```python
from build123d import *

# Parameters (mm, degrees)
BOSS_EXTRUDE1_DEPTH  = 1
SKETCH2_W            = 16
SKETCH2_H            = 10
BOSS_EXTRUDE2_DEPTH  = 10
SKETCH3_W            = 4.889113018
SKETCH3_H            = 5.37802432
CUT_EXTRUDE1_DEPTH   = 10
SKETCH4_W            = 45
SKETCH4_H            = 2.4
SKETCH4_W_2          = 30
BOSS_EXTRUDE3_DEPTH  = 4
SKETCH5_W            = 35
SKETCH5_H            = 10
BOSS_EXTRUDE4_DEPTH  = 7
SKETCH6_W            = 35
SKETCH6_H            = 1.5
CUT_EXTRUDE2_DEPTH   = 4
FILLET1_R            = 1
SKETCH7_R            = 1.5
CUT_EXTRUDE3_DEPTH   = 4
SKETCH8_W            = 0.75
SKETCH8_H            = 0.75
BOSS_EXTRUDE5_DEPTH  = 6
LPATTERN1_COUNT      = 10
LPATTERN1_PITCH      = 3
SKETCH9_W            = 0.75
SKETCH9_H            = 0.75
BOSS_EXTRUDE6_DEPTH  = 6
LPATTERN2_COUNT      = 15
LPATTERN2_PITCH      = 3
SKETCH10_R           = 2.5
BOSS_EXTRUDE7_DEPTH  = 6
SKETCH11_W           = 4.8
SKETCH11_H           = 9
BOSS_EXTRUDE8_DEPTH  = 4
SKETCH12_W           = 0.75
SKETCH12_H           = 0.75
BOSS_EXTRUDE9_DEPTH  = 6
LPATTERN3_COUNT      = 3
LPATTERN3_PITCH      = 3
LPATTERN3_COUNT_DIR2 = 2
LPATTERN3_PITCH_DIR2 = 3
SKETCH13_W           = 14.120912951
SKETCH13_H           = 4.362558473
BOSS_EXTRUDE10_DEPTH = 4
FILLET2_R            = 1


with BuildPart() as part:
    # Sketch1 → Boss-Extrude1 (new body)
    with BuildSketch(Plane.XY):
        Polygon((22.754016647, 124.270947632), (19.754016647, 127.270947632), (-47.799898806, 127.270947632), (-47.799898806, 75.270947632), (19.754016647, 75.270947632), (19.754016647, 90.113910289), (22.754016647, 92.500164177), align=None)
    extrude(amount=-BOSS_EXTRUDE1_DEPTH)

    # Sketch2 → Boss-Extrude2 (add)
    with BuildSketch(Plane(origin=(0, 0, -1), x_dir=(-1, 0, 0), z_dir=(0, 0, -1))):
        with Locations((46.316496684, 91.208096568)):
            Rectangle(SKETCH2_W, SKETCH2_H)
    extrude(amount=BOSS_EXTRUDE2_DEPTH)

    # Sketch3 → Cut-Extrude1 (cut)
    with BuildSketch(Plane.ZY.offset(54.316496684)):
        with Locations((-6.06540843, 91.2419286)):
            Rectangle(SKETCH3_W, SKETCH3_H)
    extrude(amount=-CUT_EXTRUDE1_DEPTH, mode=Mode.SUBTRACT)

    # Sketch4 → Boss-Extrude3 (add)
    with BuildSketch(Plane(origin=(0, 0, -1), x_dir=(-1, 0, 0), z_dir=(0, 0, -1))):
        with Locations((5.745983353, 78.470947632)):
            Rectangle(SKETCH4_W, SKETCH4_H)
        with Locations((-0.254016647, 124.070947632)):
            Rectangle(SKETCH4_W_2, SKETCH4_H)
    extrude(amount=BOSS_EXTRUDE3_DEPTH)

    # Sketch5 → Boss-Extrude4 (add)
    with BuildSketch(Plane(origin=(0, 0, -1), x_dir=(-1, 0, 0), z_dir=(0, 0, -1))):
        with Locations((3.745983353, 113.370947632)):
            Rectangle(SKETCH5_W, SKETCH5_H)
    extrude(amount=BOSS_EXTRUDE4_DEPTH)

    # Sketch6 → Cut-Extrude2 (cut)
    with BuildSketch(Plane(origin=(0, 0, -8), x_dir=(-1, 0, 0), z_dir=(0, 0, -1))):
        with Locations((3.745983353, 117.620947632)):
            Rectangle(SKETCH6_W, SKETCH6_H)
        with Locations((3.745983353, 109.120947632)):
            Rectangle(SKETCH6_W, SKETCH6_H)
    extrude(amount=-CUT_EXTRUDE2_DEPTH, mode=Mode.SUBTRACT)

    # Fillet1
    fillet1_edges = [part.edges().sort_by_distance(p)[0] for p in [
        (13.754016647, 109.870947632, -6),
        (-21.245983353, 109.870947632, -6),
        (13.754016647, 116.870947632, -6),
        (-21.245983353, 116.870947632, -6),
    ]]
    fillet(fillet1_edges, radius=FILLET1_R)

    # Sketch7 → Cut-Extrude3 (cut)
    with BuildSketch(Plane(origin=(0, 0, -1), x_dir=(-1, 0, 0), z_dir=(0, 0, -1))):
        with Locations((-20.390504743, 123.506772987)):
            Circle(SKETCH7_R)
        with Locations((-20.390504743, 93.48031176)):
            Circle(SKETCH7_R)
        with Locations((31.799898806, 123.506772987)):
            Circle(SKETCH7_R)
        with Locations((31.799898806, 78.192140702)):
            Circle(SKETCH7_R)
    extrude(amount=-CUT_EXTRUDE3_DEPTH, mode=Mode.SUBTRACT)

    # Sketch8 → Boss-Extrude5 (add)
    with BuildSketch(Plane(origin=(0, 0, -5), x_dir=(-1, 0, 0), z_dir=(0, 0, -1))):
        with Locations((-13.879016647, 124.070947632)):
            Rectangle(SKETCH8_W, SKETCH8_H)
    boss_extrude5 = extrude(amount=BOSS_EXTRUDE5_DEPTH)

    # LPattern1: Boss-Extrude5 ×10
    with Locations(*[(-i * LPATTERN1_PITCH, 0, 0) for i in range(1, LPATTERN1_COUNT)]):
        add(boss_extrude5)

    # Sketch9 → Boss-Extrude6 (add)
    with BuildSketch(Plane(origin=(0, 0, -5), x_dir=(-1, 0, 0), z_dir=(0, 0, -1))):
        with Locations((-15.402792453, 78.470947632)):
            Rectangle(SKETCH9_W, SKETCH9_H)
    boss_extrude6 = extrude(amount=BOSS_EXTRUDE6_DEPTH)

    # LPattern2: Boss-Extrude6 ×15
    with Locations(*[(-i * LPATTERN2_PITCH, 0, 0) for i in range(1, LPATTERN2_COUNT)]):
        add(boss_extrude6)

    # Sketch10 → Boss-Extrude7 (add)
    with BuildSketch(Plane(origin=(0, 0, -1), x_dir=(-1, 0, 0), z_dir=(0, 0, -1))):
        with Locations(Location((26.546732083, 118.214976991, 0), (0, 0, 180))):
            Circle(SKETCH10_R)
        with Locations(Location((31.940661119, 118.214976991, 0), (0, 0, 180))):
            Circle(SKETCH10_R)
    extrude(amount=BOSS_EXTRUDE7_DEPTH)

    # Sketch11 → Boss-Extrude8 (add)
    with BuildSketch(Plane(origin=(0, 0, -1), x_dir=(-1, 0, 0), z_dir=(0, 0, -1))):
        with Locations((-19.349242758, 100.613910289)):
            Rectangle(SKETCH11_W, SKETCH11_H)
    extrude(amount=BOSS_EXTRUDE8_DEPTH)

    # Sketch12 → Boss-Extrude9 (add)
    with BuildSketch(Plane(origin=(0, 0, -5), x_dir=(-1, 0, 0), z_dir=(0, 0, -1))):
        with Locations((-20.624242758, 97.488910289)):
            Rectangle(SKETCH12_W, SKETCH12_H)
    boss_extrude9 = extrude(amount=BOSS_EXTRUDE9_DEPTH)

    # LPattern3: Boss-Extrude9 3 × 2
    with Locations(*[(-j * LPATTERN3_PITCH_DIR2, i * LPATTERN3_PITCH, 0) for i in range(LPATTERN3_COUNT) for j in range(LPATTERN3_COUNT_DIR2) if (i, j) != (0, 0)]):
        add(boss_extrude9)

    # Sketch13 → Boss-Extrude10 (add)
    with BuildSketch(Plane(origin=(0, 0, -1), x_dir=(-1, 0, 0), z_dir=(0, 0, -1))):
        with Locations((23.447660741, 101.747194556)):
            Rectangle(SKETCH13_W, SKETCH13_H)
    extrude(amount=BOSS_EXTRUDE10_DEPTH)

    # Fillet2
    fillet2_edges = [part.edges().sort_by_distance(p)[0] for p in [
        (-16.387204265, 103.928473792, -3),
        (-16.387204265, 99.565915319, -3),
        (-30.508117216, 99.565915319, -3),
        (-30.508117216, 103.928473792, -3),
    ]]
    fillet(fillet2_edges, radius=FILLET2_R)


solid = part.part
```
Check sheet for the modelled part. Datum: model origin and axes. Units: mm. A direction names the side the tool comes from. Round coordinates to 2 decimals unless told otherwise and drop trailing zeros. Order: outer loops, then holes, each group sorted by start corner. A loop starts at its lowest first (then second) coordinate and runs counter-clockwise, first axis right, second up. Notation, with made-up numbers: (21, 2) -> (52, 2) arc R31 cw to (52, 32) -> close; hole circle Ø8 at (47.25, -13.75). An arc over 180 degrees is marked (long way). Use CSV: the item, a comma, the result in double quotes.
(1) Draft check along Y on faces 4 (the face through (21.23, 91.29, -0.49)), 5 (the face through (-49, 93.931, -6)), 6 (the face through (-46, 91, -11)). Enter one of: pulls with the +Y half, pulls with the -Y half, needs draft (parallel to the pull), parting line crosses it, or undercut.
Worked out:
face 4,"pulls with the -Y half"
face 5,"undercut"
face 6,"needs draft"
(2) Cross-section at B-B (z = -2). Count the separate pieces of the cut face and the enclosed holes in it, and give its area (3 significant figures).
Worked out:
separate pieces,"8"
enclosed holes,"0"
area,"833 mm²"
(3) Depth check by flat-ended pin: pin 1 (2 mm diameter, centred on x = -28, z = -3, fed in from -Y); pin 2 (1.5 mm diameter, centred on y = 112, z = -7.5, fed in from -X); pin 3 (0.6 mm diameter, centred on x = 17.5, z = -9, fed in from +Y). Enter the tip coordinate at first touch or a pass-through.
Worked out:
pin 1,"y = 77.27"
pin 2,"x = -21.25"
pin 3,"y = 103.86"
(4) Material ranges on line 1 along Y through (x, z) = (-18.5, -1.75); line 2 along Y through (x, z) = (-27, -3.25); line 3 along X through (y, z) = (97.5, -8.75), recorded low to high. Write a range as from..to.
Worked out:
line 1,"77.27..79.67, 99.57..103.93, 108.37..118.37"
line 2,"77.27..79.67, 99.57..103.93, 115.76..120.67"
line 3,"17.25..18, 20.25..21"
(5) Tool access check on faces 1 (the face through (-23, 103.928, -3)), 2 (the face through (-4, 109.871, -6)), 3 (the face through (-28.246, 78, -3)). Record the directions out of +Z, -Z, +X, -X, +Y, -Y that give a thin tool (end or side, any length) a straight path to the whole face; none if there is none.
Worked out:
face 1,"-Z, -X"
face 2,"-Z, +X, -X"
face 3,"-Z, -X, -Y"
(6) Cross-section at A-A (x = -46). Record the boundary of the cut face in (y, z).
Worked out:
outline,"(75.27, -1) -> (86.21, -1) -> (86.21, -11) -> (96.21, -11) -> (96.21, -1) -> (127.27, -1) -> (127.27, 0) -> (75.27, 0) -> close; hole (88.55, -8.51) -> (93.93, -8.51) -> (93.93, -3.62) -> (88.55, -3.62) -> close"
(7) Cross-section at D-D (y = 106). Record the boundary of the cut face in (x, z), and give its area (3 significant figures).
Worked out:
outline,"(-47.8, -1) -> (22.75, -1) -> (22.75, 0) -> (-47.8, 0) -> close"
area,"70.6 mm²"
